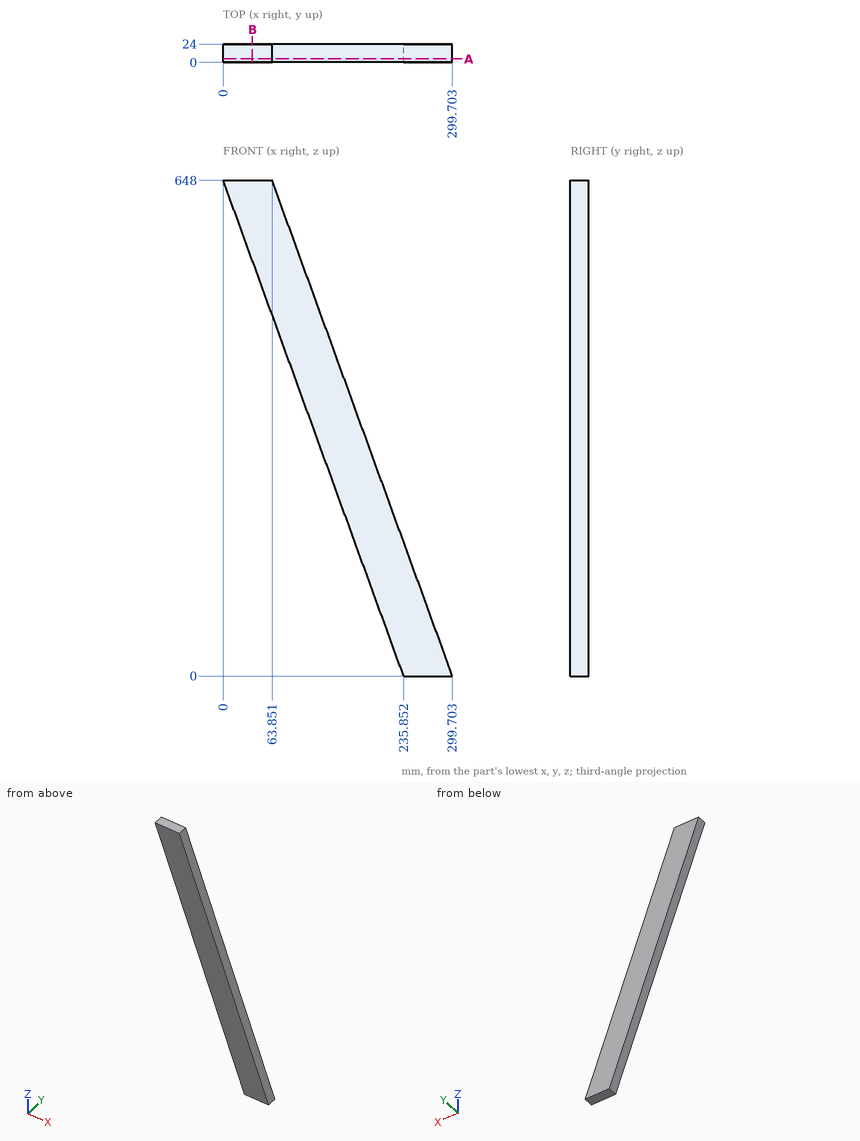
Answer from the drawing. Dimensions are ordinates in mm from the lowest x, y and z of the part. Round coordinates to 2 decimals unless told otherwise and drop trailing zeros. Loops run counter-clockwise (first coordinate to the right, second up) from the corner with the lowest first, then second, coordinate; pieces in that order, holes last.
1) Given P1, Ø12, axis at y = 11.5, z = 544, coming from the -X side; P2, Ø2, axis at y = 9, z = 119, coming from the -X side, each flat-ended and moving along its own axis, determine where each tip first touches the part or whether it passes through.
Outcome:
P1: stops at x = 35.67
P2: stops at x = 192.18
2) Consider line 1 (X direction, y = 5, z = 515); line 2 (X direction, y = 6.25, z = 572). Determine where each line is inside the solid, lowest interval first.
Outcome:
line 1: x = 48.41 to 112.26
line 2: x = 27.66 to 91.51
3) A cutting plane is placed at A-A on y = 4.5. Determine the outline of the cut face in (x, z).
Outcome:
outline: (0, 648) - (235.85, 0) - (299.7, 0) - (63.85, 648) - close
4) A cutting plane is placed at B-B on x = 38. Determine the outline of the cut face in (y, z) (1 decimal), plus the area to 3 significant figures.
Outcome:
outline: (0, 543.6) - (24, 543.6) - (24, 648) - (0, 648) - close
area: 2,510 mm2
